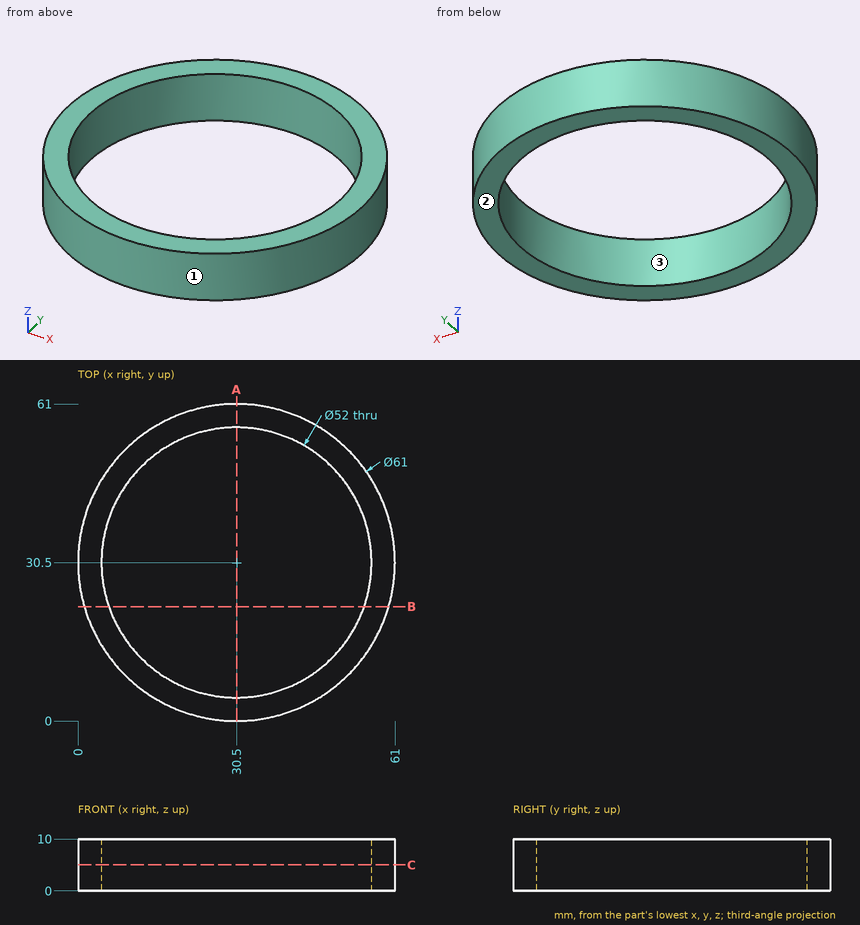
The figure shows three views and two pictorial views of one solid part (mm, origin at its lowest corner). Answer the questions. Round coordinates to 2 decimals unless told otherwise and drop trailing zeros. Write each loop counter-clockwise with the first axis right and the second up, starting at its lowest first coordinate (ties: lowest second). Pieces come first, ordered by that corner, then holes. Notation, with made-up numbers: (14.5, -33) -> (20.5, -33) arc R14 cw to (20.5, -10) -> close; hole circle Ø1 at (89.5, 1). An arc over 180 degrees is marked (long way). Write each question's results on one line, items separated by ' | '.
Q1. Section C-C, the plane z = 5 is taken. Write down the section's boundary in (x, y), then the cut area to 3 significant figures.
Data:
outline: circle Ø61 at (30.5, 30.5); hole circle Ø52 at (30.5, 30.5) | area: 799 mm^2
Q2. Flat-ended cylindrical pins translate along their axes: P1, Ø6, axis at x = 46.5, z = 3.5, coming from the +Y side; P2, Ø4, axis at x = 10, z = 3, coming from the -Y side; P3, Ø4, axis at y = 51.5, z = 4.5, coming from the +X side. Find the tip coordinate at first contact, or state that the pin passes through.
Data:
P1: y = 58.09 | P2: y = 6.25 | P3: x = 54.36
Q3. Section B-B, the plane y = 22 is taken. Write down the section's boundary in (x, z).
Data:
outline: (1.21, 0) -> (5.93, 0) -> (5.93, 10) -> (1.21, 10) -> close; (55.07, 0) -> (59.79, 0) -> (59.79, 10) -> (55.07, 10) -> close
Q4. Determine the mould class of the marked faces 1, 2 and 3 for opening direction X: released by +X, released by -X, zero draft, split by the parting line, or undercut.
Data:
face 1: split by the parting line | face 2: zero draft | face 3: undercut
Q5. Section A-A, the plane x = 30.5 is taken. Write down the section's boundary in (y, z).
Data:
outline: (0, 0) -> (4.5, 0) -> (4.5, 10) -> (0, 10) -> close; (56.5, 0) -> (61, 0) -> (61, 10) -> (56.5, 10) -> close
Q6. Straight lines are drawn through the part: line 1 along Y through (x, z) = (30.5, 2.5); line 2 along X through (y, z) = (47, 2); line 3 along X through (y, z) = (6.5, 9.5). For each, find the intervals that lie inside material, in ascending order. Write a range as [from, to].
Data:
line 1: [0, 4.5], [56.5, 61] | line 2: [4.85, 10.41], [50.59, 56.15] | line 3: [11.68, 20.5], [40.5, 49.32]
